```python
from build123d import *

# Parameters (mm, degrees)
SKETCH1_R                  = 50
BOSS_EXTRUDE1_DEPTH        = 5
F_15_0_15_DIAMETER_HOLE1_D = 15
F_14_0_14_DIAMETER_HOLE1_D = 14
SKETCH9_R                  = 2
CUT_EXTRUDE1_DEPTH         = 10
SKETCH10_R                 = 6
CUT_EXTRUDE2_DEPTH         = 10
SKETCH11_R                 = 1.5
CUT_EXTRUDE3_DEPTH         = 10
SKETCH12_R                 = 1.5
CUT_EXTRUDE4_DEPTH         = 10
SKETCH13_R                 = 1.5
CUT_EXTRUDE5_DEPTH         = 10
SKETCH14_R                 = 4
CUT_EXTRUDE6_DEPTH         = 10
CUT_EXTRUDE7_DEPTH         = 10


with BuildPart() as part:
    # Sketch1 → Boss-Extrude1 (new body)
    with BuildSketch(Plane.XY):
        Circle(SKETCH1_R)
    extrude(amount=BOSS_EXTRUDE1_DEPTH)

    # Ø15.0 (15) Diameter Hole1 (through all)
    with Locations(Plane(origin=(0, 0, 0), x_dir=(-1, 0, 0), z_dir=(0, 0, -1))):
        with Locations((0, 0)):
            Hole(F_15_0_15_DIAMETER_HOLE1_D / 2)

    # Ø14.0 (14) Diameter Hole1 (through all)
    with Locations(Plane(origin=(0, 0, 0), x_dir=(-1, 0, 0), z_dir=(0, 0, -1))):
        with Locations((37, 0), (-37, 0)):
            Hole(F_14_0_14_DIAMETER_HOLE1_D / 2)

    # Sketch9 → Cut-Extrude1 (cut)
    with BuildSketch(Plane.XY.offset(5)):
        with Locations((12.5, 5.5)):
            Circle(SKETCH9_R)
        with Locations((12.5, -12.5)):
            Circle(SKETCH9_R)
        with Locations((-12.5, -12.5)):
            Circle(SKETCH9_R)
        with Locations((-12.5, 5.5)):
            Circle(SKETCH9_R)
    extrude(amount=-CUT_EXTRUDE1_DEPTH, mode=Mode.SUBTRACT)

    # Sketch10 → Cut-Extrude2 (cut)
    with BuildSketch(Plane.XY.offset(5)):
        with Locations((0, -40)):
            Circle(SKETCH10_R)
    extrude(amount=-CUT_EXTRUDE2_DEPTH, mode=Mode.SUBTRACT)

    # Sketch11 → Cut-Extrude3 (cut)
    with BuildSketch(Plane.XY.offset(5)):
        with Locations((30.0520382, -18.03122292)):
            Circle(SKETCH11_R)
        with Locations((30.0520382, -30.0520382)):
            Circle(SKETCH11_R)
        with Locations((18.03122292, -30.0520382)):
            Circle(SKETCH11_R)
        with Locations((18.03122292, -18.03122292)):
            Circle(SKETCH11_R)
    cut_extrude3 = extrude(amount=-CUT_EXTRUDE3_DEPTH, mode=Mode.SUBTRACT)

    # Mirror1: Cut-Extrude3 across plane
    add(cut_extrude3.mirror(Plane(origin=(0, 0, 0), x_dir=(0, 0, 1), z_dir=(1, 0, 0))), mode=Mode.SUBTRACT)

    # Sketch12 → Cut-Extrude4 (cut)
    with BuildSketch(Plane.XY.offset(5)):
        with Locations((6.01040764, 40.01040764)):
            Circle(SKETCH12_R)
        with Locations((6.01040764, 27.98959236)):
            Circle(SKETCH12_R)
        with Locations((-6.01040764, 27.98959236)):
            Circle(SKETCH12_R)
        with Locations((-6.01040764, 40.01040764)):
            Circle(SKETCH12_R)
    extrude(amount=-CUT_EXTRUDE4_DEPTH, mode=Mode.SUBTRACT)

    # Sketch13 → Cut-Extrude5 (cut)
    with BuildSketch(Plane.XY.offset(5)):
        with Locations((-47, 0)):
            Circle(SKETCH13_R)
        with Locations((-27, 0)):
            Circle(SKETCH13_R)
        with Locations((-10, -40)):
            Circle(SKETCH13_R)
        with Locations((10, -40)):
            Circle(SKETCH13_R)
        with Locations((27, 0)):
            Circle(SKETCH13_R)
        with Locations((47, 0)):
            Circle(SKETCH13_R)
    extrude(amount=-CUT_EXTRUDE5_DEPTH, mode=Mode.SUBTRACT)

    # Sketch14 → Cut-Extrude6 (cut)
    with BuildSketch(Plane.XY.offset(5)):
        with Locations((28.284271247, 28.284271247)):
            Circle(SKETCH14_R)
    extrude(amount=-CUT_EXTRUDE6_DEPTH, mode=Mode.SUBTRACT)

    # Sketch15 → Cut-Extrude7 (cut)
    with BuildSketch(Plane.XY.offset(5)):
        with BuildLine():
            Line((-17.012303521, 38.933386687), (-16.280949819, 38.251388327))
            ThreePointArc((-16.280949819, 38.251388327), (-15.646164885, 36.858479918), (-16.182239136, 35.424684204))
            Line((-16.182239136, 35.424684204), (-37.324188298, 12.752719454))
            ThreePointArc((-37.324188298, 12.752719454), (-38.717096708, 12.11793452), (-40.150892422, 12.654008771))
            Line((-40.150892422, 12.654008771), (-40.882246123, 13.336007131))
            ThreePointArc((-40.882246123, 13.336007131), (-41.517031057, 14.728915541), (-40.980956806, 16.162711254))
            Line((-40.980956806, 16.162711254), (-19.839007644, 38.834676004))
            ThreePointArc((-19.839007644, 38.834676004), (-18.446099234, 39.469460938), (-17.012303521, 38.933386687))
        make_face()
    extrude(amount=-CUT_EXTRUDE7_DEPTH, mode=Mode.SUBTRACT)


solid = part.part
```
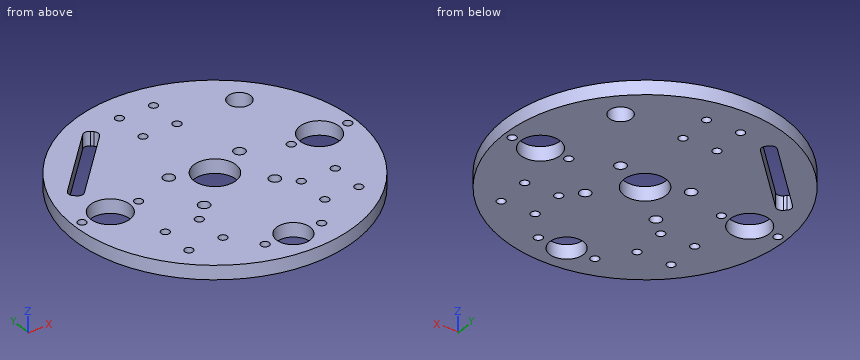
Check sheet for the modelled part. Datum: model origin and axes. Units: mm. Coordinates: 2 decimals unless noted, no trailing zeros. Loops run counter-clockwise (first coordinate to the right, second up) from the corner with the lowest first, then second, coordinate; pieces in that order, holes last.
1) Sectioned sample at A-A (x = 0). Record the boundary of the cut face in (y, z).
2) Gauge pin test, flat end, axial feed: pin 1 (1 mm diameter, centred on y = -10.5, z = 2, fed in from -X). Record the tip position at first contact, or that the pin passes through.
3) Material ranges on probe 1 along Y at (x, z) = (17, 2); probe 2 along Y at (x, z) = (1.5, 1.15); probe 3 along X at (y, z) = (-14, 0.5), recorded low to high.
4) Sectioned sample at D-D (y = -12.5). Record the boundary of the cut face in (x, z), and give its area (3 significant figures).
5) Sectioned sample at C-C (x = 38). Record the boundary of the cut face in (y, z).
6) Sectioned sample at B-B (y = 0). Count the separate pieces of the cut face and the enclosed holes in it, and give its area (3 significant figures).
Check sheet entries:
1. outline: (-50, 0) - (-46, 0) - (-46, 5) - (-50, 5) - close; (-34, 0) - (-7.5, 0) - (-7.5, 5) - (-34, 5) - close; (7.5, 0) - (50, 0) - (50, 5) - (7.5, 5) - close
2. pin 1: stops at x = -48.99
3. probe 1: y = -47.02 to -31.14, -28.96 to -19.12, -16.94 to 47.02
3. probe 2: y = -49.98 to -45.81, -34.19 to -7.35, 7.35 to 49.98
3. probe 3: x = -48 to -13.82, -11.18 to 11.18, 13.82 to 48
4. outline: (-48.41, 0) - (-14.5, 0) - (-14.5, 5) - (-48.41, 5) - close; (-10.5, 0) - (10.5, 0) - (10.5, 5) - (-10.5, 5) - close; (14.5, 0) - (48.41, 0) - (48.41, 5) - (14.5, 5) - close
4. area: 444 mm2
5. outline: (-32.5, 0) - (-6.93, 0) - (-6.93, 5) - (-32.5, 5) - close; (6.93, 0) - (32.5, 0) - (32.5, 5) - (6.93, 5) - close
6. separate pieces: 8
6. enclosed holes: 0
6. area: 225 mm2
